from build123d import *

# Parameters (mm, degrees)
SALIENTE_EXTRUIR1_DEPTH = 3
SALIENTE_EXTRUIR2_DEPTH = 7
CROQUIS3_R              = 2
CORTAR_EXTRUIR1_DEPTH   = 91.19977827
CHAFL_N1_SIZE           = 3


with BuildPart() as part:
    # Croquis1 → Saliente-Extruir1 (new body)
    with BuildSketch(Plane(origin=(0, 0, 0), x_dir=(1, 0, 0), z_dir=(0, 1, 0))):
        Polygon((-15, -10), (15, -10), (60, -28), (70, -28), (70, 28), (60, 28), (15, 10), (-15, 10), align=None)
    extrude(amount=SALIENTE_EXTRUIR1_DEPTH)

    # Croquis2 → Saliente-Extruir2 (add)
    with BuildSketch(Plane(origin=(0, 3, 0), x_dir=(1, 0, 0), z_dir=(0, 1, 0))):
        Polygon((-15, 10), (15, 10), (60, 28), (70, 28), (70, 26), (60, 26), (15, 8), (-15, 8), align=None)
        Polygon((-15, -10), (15, -10), (60, -28), (70, -28), (70, -26), (60, -26), (15, -8), (-15, -8), align=None)
    extrude(amount=SALIENTE_EXTRUIR2_DEPTH)

    # Croquis3 → Cortar-Extruir1 (cut, through all)
    with BuildSketch(Plane.XY.offset(28)):
        with Locations((65, 7)):
            Circle(CROQUIS3_R)
    extrude(amount=-CORTAR_EXTRUIR1_DEPTH, mode=Mode.SUBTRACT)

    # Chaflán1
    chafl_n1_edges = [part.edges().sort_by_distance(p)[0] for p in [
        (70, 10, -27),
        (70, 10, 27),
    ]]
    chamfer(chafl_n1_edges, length=CHAFL_N1_SIZE)


solid = part.part
Geometry check sheet. Reference: the model listing, model coordinates, mm. A direction names the side the tool comes from. Round coordinates to 2 decimals unless told otherwise and drop trailing zeros. Order: outer loops, then holes, each group sorted by start corner. A loop starts at its lowest first (then second) coordinate and runs counter-clockwise, first axis right, second up. Notation, with made-up numbers: M -9,-17.75 L 30,-17.75 A27 cw 30,20.25 Z; hole C 30,29.25 d6. An arc over 180 degrees is marked long. Write each question's results on one line, items separated by ' | '. Start each with the question number.
1. Cross-section at A-A on x = 65. Record the boundary of the cut face in (y, z), plus the area to 3 significant figures.
2. Material ranges on L1, parallel to Y at x = 65, z = 27; L2, parallel to Z at x = -11.5, y = 6.5; L3, parallel to Z at x = 63, y = 6.5, recorded low to high. Write a range as from..to.
3. Set-up check for faces 4 (the face through (36, 0, 0)), 5 (the face through (68, 9, 27)), 6 (the face through (36, 3, 0)), 7 (the face through (0, 5, -10)), 8 (the face through (0, 6, 8)): record each of +Z, -Z, +X, -X, +Y, -Y from which the full face is reachable in a straight line by a thin tool's end or side.
4. Cross-section at C-C on x = 26. Record the boundary of the cut face in (y, z), plus the area to 3 significant figures.
5. Draft check along Y on faces 1 (the face through (63.526, 8.352, 27.014)), 2 (the face through (70, 1, 0)), 3 (the face through (26, 10, 14)). Enter one of: pulls with the +Y half, pulls with the -Y half, needs draft (parallel to the pull), parting line crosses it, or undercut.
6. Go/stop test with flat-tipped pins: P1, Ø4, axis at x = 52, z = 9, coming from the +Y side; P2, Ø3.5, axis at x = 6, y = 5, coming from the -Z side; P3, Ø5, axis at x = -4.5, y = 6, coming from the +Z side; P4, Ø6, axis at x = 2, z = 0, coming from the -Y side. Record where each tip stops, or that it passes through.
7. Cross-section at B-B on y = 1. Record the boundary of the cut face in (x, z).
8. Cross-section at D-D on z = -23. Record the boundary of the cut face in (x, y).
Resolved:
1) outline: M 0,-28 L 5,-28 L 5,-26 L 3,-26 L 3,26 L 5,26 L 5,28 L 0,28 Z; M 9,-28 L 10,-28 L 10,-26 L 9,-26 Z; M 9,26 L 10,26 L 10,28 L 9,28 Z | area: 180 mm2
2) L1: 0..5, 9..10 | L2: -10..-8, 8..10 | L3: -28..-26, 26..28
3) face 4: +Z, -Z, +X, -X, -Y | face 5: +Z, -Z, +X, +Y | face 6: +X, +Y | face 7: -Z, -X, +Y, -Y | face 8: +X, -X, +Y
4) outline: M 0,-14.4 L 10,-14.4 L 10,-12.4 L 3,-12.4 L 3,12.4 L 10,12.4 L 10,14.4 L 0,14.4 Z | area: 114 mm2
5) face 1: undercut | face 2: needs draft | face 3: pulls with the +Y half
6) P1: y = 3 | P2: z = -10 | P3: z = 10 | P4: y = 0
7) outline: M -15,-10 L 15,-10 L 60,-28 L 70,-28 L 70,28 L 60,28 L 15,10 L -15,10 Z
8) outline: M 47.5,0 L 70,0 L 70,3 L 52.5,3 L 52.5,10 L 47.5,10 Z
